Answer from the drawing. Dimensions are ordinates in mm from the lowest x, y and z of the part. A direction names the side the tool comes from. Coordinates: 2 decimals unless noted, no trailing zeros. Write each loop counter-clockwise with the first axis right and the second up, starting at its lowest first coordinate (ties: lowest second). Pieces come first, ordered by that corner, then holes.
(1) The part is cut by section B-B, the plane x = 10. Determine the outline of the cut face in (y, z), and give its area (3 significant figures).
(2) Which of the six approach directions +Z, -Z, +X, -X, +Y, -Y give full straight-line access (tool end or side, diameter ignored) to the marked faces 4 and 5?
(3) Determine the mould class of the marked faces 1, 2 and 3 for opening direction X: pulls with the +X half, pulls with the -X half, needs draft (parallel to the pull), parting line crosses it, or undercut.
(4) The part is cut by section C-C, the plane y = 25.75. Determine the outline of the cut face in (x, z).
(5) The part is cut by section A-A, the plane y = 19.75. Determine the outline of the cut face in (x, z), and give its area (3 significant figures).
(6) Straight lines are drawn through the part: line 1 along X through (y, z) = (5, 11.75); line 2 along Z through (x, y) = (130, 17); line 3 along X through (y, z) = (19.5, 8.25) (1 decimal). For each, find the intervals that lie inside material, in ascending order.
(7) The part is cut by section D-D, the plane x = 81. Determine the outline of the cut face in (y, z).
(8) Given pin 1 (3 mm diameter, centred on x = 10, z = 10, fed in from -Y); pin 2 (6 mm diameter, centred on x = 72.5, z = 9, fed in from +Y); pin 3 (4.5 mm diameter, centred on x = 93.5, z = 10, fed in from +Y); pin 4 (3 mm diameter, centred on x = 94, z = 10, fed in from -Y), each flat-ended and moving along its own axis, determine where each tip first touches the part or whether it passes through.
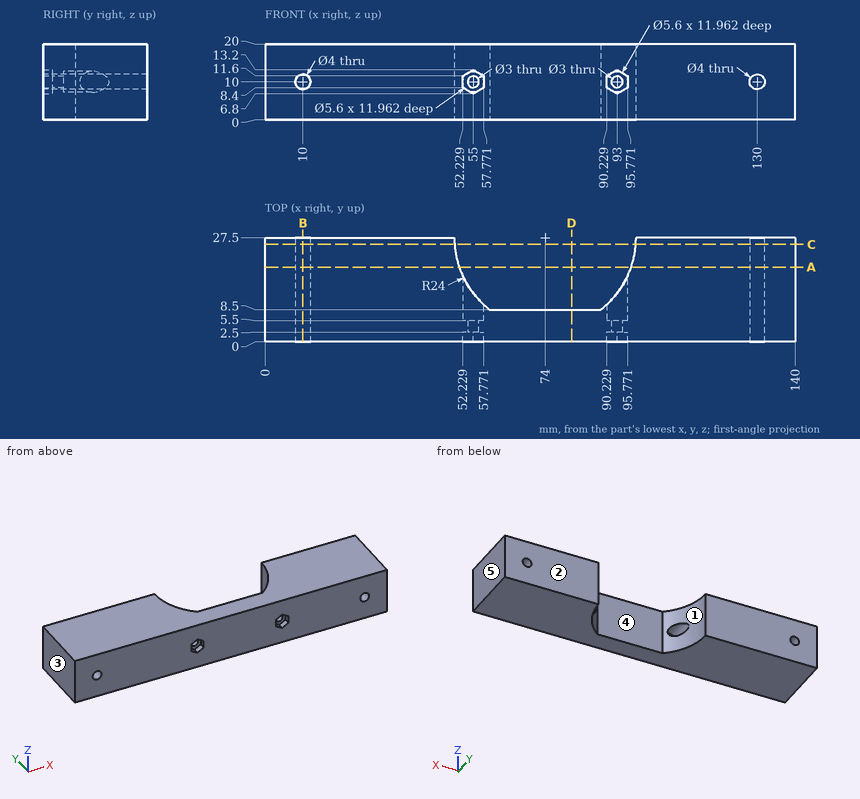
Computed:
1. outline: (0, 0) - (27.5, 0) - (27.5, 8) - (0, 8) - close; (0, 12) - (27.5, 12) - (27.5, 20) - (0, 20) - close
1. area: 440 mm2
2. face 4: +Z, -Z, +Y
2. face 5: +Z, -Z, +X, +Y, -Y
3. face 1: undercut
3. face 2: needs draft
3. face 3: pulls with the -X half
4. outline: (0, 0) - (50.06, 0) - (50.06, 20) - (0, 20) - close; (97.94, 0) - (140, 0) - (140, 20) - (97.94, 20) - close; hole circle Ø4 at (10, 10); hole circle Ø4 at (130, 10)
5. outline: (0, 0) - (51.29, 0) - (51.29, 20) - (0, 20) - close; (96.71, 0) - (140, 0) - (140, 20) - (96.71, 20) - close; hole circle Ø4 at (10, 10); hole circle Ø4 at (130, 10)
5. area: 1,870 mm2
6. line 1: x = 0 to 9.03, 10.97 to 129.03, 130.97 to 140
6. line 2: z = 0 to 8, 12 to 20
6. line 3: x = 0 to 9, 11 to 51.4, 96.6 to 129, 131 to 140
7. outline: (0, 0) - (8.5, 0) - (8.5, 20) - (0, 20) - close
8. pin 1: passes through
8. pin 2: stops at y = 8.5
8. pin 3: stops at y = 5.5
8. pin 4: stops at y = 2.5
